Autodesk Inventor part; units mm, degrees
ref_plane "YZ Plane" through (0, 0, 0) normal (1, 0, 0) x (0, 1, 0)
ref_plane "XZ Plane" through (0, 0, 0) normal (0, 1, 0) x (-1, 0, 0)
ref_plane "XY Plane" through (0, 0, 0) normal (0, 0, 1) x (1, 0, 0)
ref_plane "작업 평면1" through (23.5, -8, -2) normal (1, 0, 0) x (0, 0, -1)
sketch "스케치1" plane through (23.5, -8, -2) normal (1, 0, 0) x (0, 0, -1)
  line L0 (0, 16) -> (-8.15, 16)
  line L1 (-8.15, 16) -> (-8.15, 10.6)
  line L2 (-8.15, 10.6) -> (-12.15, 10.6)
  line L3 (-13.15, 9.6) -> (-12.15, 10.6)
  line L4 (-13.15, 9.6) -> (-13.15, 6.4)
  line L5 (-12.15, 5.4) -> (-13.15, 6.4)
  line L6 (-12.15, 5.4) -> (-8.15, 5.4)
  line L7 (-8.15, 5.4) -> (-8.15, 0)
  line L8 (-8.15, 0) -> (0, 0)
  line L9 (0, 16) -> (6.35, 16)
  line L10 (6.35, 16) -> (6.35, 15)
  line L11 (4.35, 14) -> (4.35, 2)
  line L12 (4.35, 14) -> (5.35, 14)
  line L13 (0, 0) -> (6.35, 0)
  line L14 (6.35, 0) -> (6.35, 1)
  line L15 (4.35, 2) -> (5.35, 2)
  line L16 (0, 16) -> (-8.15, 16)
  line L17 (-8.15, 10.6) -> (-12.15, 10.6)
  line L18 (-8.15, 10.6) -> (-12.15, 10.6)
  line L19 (-12.15, 10.6) -> (-13.15, 9.6)
  line L20 (-13.15, 6.4) -> (-12.15, 5.4)
  line L21 (5.35, 14) -> (6.35, 14)
  line L22 (6.35, 14) -> (6.35, 15)
  line L23 (5.35, 2) -> (6.35, 2)
  line L24 (6.35, 2) -> (6.35, 1)
  point P0 (-2, 8)
  dimension "d1" = 6.35
sketch "스케치2" plane through (-23.5, 8, 6.15) normal (0, 0, 1) x (1, 0, 0)
  arc A0 (7.9209, -9.6) -> (7.9209, -6.4) centre (6, -8) ccw
  line L0 (39.0791, -9.6) -> (7.9209, -9.6)
  circle A1 centre (6, -8) radius 2.5
  circle A2 centre (41, -8) radius 2.5
  circle A3 centre (41, -8) radius 2.5
  point P0 (23.5, -8)
  point P1 (7.9209, -6.4)
extrude "돌출1" add sketch "스케치1" against normal up to surface (47 mm away)
extrude "돌출2" cut sketch "스케치2" along normal mid plane 50
sketch "스케치3" plane through (-15.5791, 1.6, 11.15) normal (0, 0, 1) x (1, 0, 0)
  line L0 (15.5791, -14.4593) -> (15.5791, 15.5737)
  line L1 (-7.9209, 4.4) -> (-7.9209, -7.6)
  line L2 (-7.9209, 4.4) -> (11.0791, 4.4)
  line L3 (11.0791, 4.4) -> (11.0791, -7.6)
  line L4 (11.0791, -7.6) -> (-7.9209, -7.6)
  line L5 (-7.9209, -7.6) -> (-7.9209, 4.4)
  line L6 (39.0791, 4.4) -> (39.0791, -7.6)
  line L7 (39.0791, 4.4) -> (20.0791, 4.4)
  line L8 (20.0791, 4.4) -> (20.0791, -7.6)
  line L9 (20.0791, -7.6) -> (39.0791, -7.6)
  line L10 (39.0791, -7.6) -> (39.0791, 4.4)
  point P0 (15.5791, -1.6)
  dimension "d9" = 19
extrude "돌출3" cut sketch "스케치3" against normal up to surface (5 mm away)
sketch "스케치4" plane through (-4.5, 1.6, 11.15) normal (0, 0, 1) x (1, 0, 0)
  line L0 (2.1691, -0.2851) -> (8.7999, -0.2851) construction
  line L1 (8.7999, -0.2851) -> (8.7999, -2.6545) construction
  line L2 (8.7999, -2.6545) -> (2.1691, -2.6545) construction
  line L3 (2.1691, -2.6545) -> (2.1691, -0.2851) construction
  spline S0 degree 2 poles (3.9352, -1.6066) (3.9352, -2.29) (3.5379, -2.9301) (3.1242, -2.9301) knots 0 0 0 1 2 2 2
  spline S1 degree 2 poles (3.1242, -2.9301) (2.7043, -2.9301) (2.3111, -2.2776) (2.3111, -1.6087) knots 0 0 0 1 2 2 2
  spline S2 degree 2 poles (2.3111, -1.6087) (2.3111, -0.9212) (2.7084, -0.2851) (3.1242, -0.2851) knots 0 0 0 1 2 2 2
  spline S3 degree 2 poles (3.1242, -0.2851) (3.542, -0.2851) (3.9352, -0.9438) (3.9352, -1.6066) knots 0 0 0 1 2 2 2
  spline S4 degree 2 poles (3.4988, -2.3805) (3.5482, -2.255) (3.5894, -1.868) (3.5894, -1.6066) knots 0 0 0 1 2 2 2
  spline S5 degree 2 poles (3.5894, -1.6066) (3.5894, -1.3452) (3.5482, -0.9603) (3.4967, -0.8306) knots 0 0 0 1 2 2 2
  spline S6 degree 2 poles (3.4967, -0.8306) (3.4453, -0.7009) (3.2662, -0.5671) (3.1242, -0.5671) knots 0 0 0 1 2 2 2
  spline S7 degree 2 poles (3.1242, -0.5671) (2.9822, -0.5671) (2.799, -0.7009) (2.7454, -0.8347) knots 0 0 0 1 2 2 2
  spline S8 degree 2 poles (2.7454, -0.8347) (2.694, -0.9644) (2.6569, -1.3596) (2.6569, -1.6087) knots 0 0 0 1 2 2 2
  spline S9 degree 2 poles (2.6569, -1.6087) (2.6569, -1.8762) (2.6899, -2.2344) (2.7434, -2.3744) knots 0 0 0 1 2 2 2
  spline S10 degree 2 poles (2.7434, -2.3744) (2.7928, -2.5061) (2.976, -2.6481) (3.1242, -2.6481) knots 0 0 0 1 2 2 2
  spline S11 degree 2 poles (3.1242, -2.6481) (3.2641, -2.6481) (3.4473, -2.5143) (3.4988, -2.3805) knots 0 0 0 1 2 2 2
  line L4 (4.8058, -2.8766) -> (4.3983, -2.8766)
  line L5 (4.3983, -2.8766) -> (4.3983, -2.3908)
  line L6 (4.3983, -2.3908) -> (4.8058, -2.3908)
  line L7 (4.8058, -2.3908) -> (4.8058, -2.8766)
  spline S12 degree 2 poles (6.8992, -1.6066) (6.8992, -2.29) (6.5019, -2.9301) (6.0882, -2.9301) knots 0 0 0 1 2 2 2
  spline S13 degree 2 poles (6.0882, -2.9301) (5.6683, -2.9301) (5.2752, -2.2776) (5.2752, -1.6087) knots 0 0 0 1 2 2 2
  spline S14 degree 2 poles (5.2752, -1.6087) (5.2752, -0.9212) (5.6724, -0.2851) (6.0882, -0.2851) knots 0 0 0 1 2 2 2
  spline S15 degree 2 poles (6.0882, -0.2851) (6.506, -0.2851) (6.8992, -0.9438) (6.8992, -1.6066) knots 0 0 0 1 2 2 2
  spline S16 degree 2 poles (6.4628, -2.3805) (6.5122, -2.255) (6.5534, -1.868) (6.5534, -1.6066) knots 0 0 0 1 2 2 2
  spline S17 degree 2 poles (6.5534, -1.6066) (6.5534, -1.3452) (6.5122, -0.9603) (6.4608, -0.8306) knots 0 0 0 1 2 2 2
  spline S18 degree 2 poles (6.4608, -0.8306) (6.4093, -0.7009) (6.2302, -0.5671) (6.0882, -0.5671) knots 0 0 0 1 2 2 2
  spline S19 degree 2 poles (6.0882, -0.5671) (5.9462, -0.5671) (5.763, -0.7009) (5.7095, -0.8347) knots 0 0 0 1 2 2 2
  spline S20 degree 2 poles (5.7095, -0.8347) (5.658, -0.9644) (5.621, -1.3596) (5.621, -1.6087) knots 0 0 0 1 2 2 2
  spline S21 degree 2 poles (5.621, -1.6087) (5.621, -1.8762) (5.6539, -2.2344) (5.7074, -2.3744) knots 0 0 0 1 2 2 2
  spline S22 degree 2 poles (5.7074, -2.3744) (5.7568, -2.5061) (5.94, -2.6481) (6.0882, -2.6481) knots 0 0 0 1 2 2 2
  spline S23 degree 2 poles (6.0882, -2.6481) (6.2282, -2.6481) (6.4114, -2.5143) (6.4628, -2.3805) knots 0 0 0 1 2 2 2
  point P0 (4.5, -1.6)
extrude "돌출4" cut sketch "스케치4" against normal blind 5
properties part number "Bearing Spacer_V2_0mm"
Read the model definition and answer for the solid it produces. Units are mm, in the model's axes. A direction names the side the tool comes from. Coordinates: 2 decimals unless noted, no trailing zeros. Order: outer loops, then holes, each group sorted by start corner. A loop starts at its lowest first (then second) coordinate and runs counter-clockwise, first axis right, second up. Notation, with made-up numbers: M 41.5,31.5 L 55.5,31.5 A17 ccw 55.5,36.5 Z; hole C 34.5,78.5 d2. An arc over 180 degrees is marked long. Put each result on its own line as item: value. Start each with the question number.
Item 1: For faces 4 (the face through (0, -2.6, 8)), 5 (the face through (-15, 0, 0)), 6 (the face through (4.5, 0, 9)), 7 (the face through (0, -6, -7)), 8 (the face through (-4.5, 0, 9)), determine the directions among +Z, -Z, +X, -X, +Y, -Y from which every point of the face is accessible in a straight line to the end or side of a thin tool.
Item 2: Section A-A, the plane x = 17.5 is taken. Determine the outline of the cut face in (y, z).
Item 3: The mould has two halves that part along Y. Classify faces 1 (the face through (0, 4, 6.15)), 2 (the face through (0, 8, -1)), 3 (the face through (-2, 0, 6.15)): +Y half, -Y half, draft (parallel to the pull), parting line (faces both ways), or undercut.
Item 4: Section B-B, the plane x = 3 is taken. Determine the outline of the cut face in (y, z).
Item 5: Consider probe 1 along Y at (x, z) = (-17.5, 2.5); probe 2 along X at (y, z) = (1.5, -1.25); probe 3 along Z at (x, y) = (13, -3.5). Determine where each line is inside the solid, lowest interval first. Write a range as [from, to].
Item 6: Section C-C, the plane z = -1 is taken. Determine the outline of the cut face in (x, y), plus the area to 3 significant figures.
Item 7: Given pin 1 Ø3.5 at (x, y) = (-1.5, 1) entering from -Z; pin 2 Ø2.5 at (y, z) = (1, 7.5) entering from +X; pin 3 Ø5 at (x, y) = (-8.5, 3.5) entering from +Z; pin 4 Ø3 at (x, y) = (-17.5, 0) entering from -Z, each flat-ended and moving along its own axis, determine where each tip first touches the part or whether it passes through.
Computed:
1. face 4: +Z, +X, -X, -Y
1. face 5: +Z, -Z
1. face 6: +Z, +X, +Y, -Y
1. face 7: -Z, +X, -X
1. face 8: +Z, -X, +Y, -Y
2. outline: M -8,-8.35 L -6,-8.35 L -6,-6.35 L -2.5,-6.35 L -2.5,6.15 L -8,6.15 Z; M 2.5,-6.35 L 6,-6.35 L 6,-8.35 L 8,-8.35 L 8,6.15 L 2.5,6.15 Z
3. face 1: draft
3. face 2: +Y half
3. face 3: undercut
4. outline: M -8,-8.35 L -6,-8.35 L -6,-6.35 L 6,-6.35 L 6,-8.35 L 8,-8.35 L 8,6.15 L 2.6,6.15 L 2.6,10.15 L 1.6,11.15 L -1.6,11.15 L -2.6,10.15 L -2.6,6.15 L -8,6.15 Z
5. probe 1: y = [-8, -2.5], [2.5, 8]
5. probe 2: x = [-23.5, -19.5], [-15.5, 15.5], [19.5, 23.5]
5. probe 3: z = [-6.35, 6.15]
6. outline: M -23.5,-8 L 23.5,-8 L 23.5,8 L -23.5,8 Z; hole C -17.5,0 d5; hole C 17.5,0 d5
6. area: 713 mm2
7. pin 1: stops at z = -6.35
7. pin 2: stops at x = 4.5
7. pin 3: stops at z = 6.15
7. pin 4: passes through
